```python
from build123d import *
from build123d import SkipClean  # not in build123d's __all__

# Parameters (mm, degrees)
F0_R      = 15
F1_DEPTH  = 67
F2_R      = 10
F3_DEPTH  = 11
F4_R      = 8.5
F5_DEPTH  = 1.9
F6_R      = 6.5
F7_DEPTH  = 2.1
F9_DEPTH  = 2
F10_W     = 1.5
F10_H     = 7
F11_DEPTH = 7
F13_DEPTH = 9.0692195411
F15_DEPTH = 25
F16_R     = 13.5
F17_DEPTH = 58.88


with BuildPart() as f1:
    # F0 (on Front) → F1 (new body)
    with BuildSketch(Plane.XZ):
        Circle(F0_R)
    extrude(amount=F1_DEPTH)

    # F2 (on face) → F3 (join)
    with BuildSketch(Plane.XZ.offset(67)):
        with Locations((-3.3, 0)):
            Circle(F2_R)
    extrude(amount=F3_DEPTH)

    # F4 (on face) → F5 (join)
    with BuildSketch(Plane.XZ.offset(78)):
        with Locations((-3.3, 0)):
            Circle(F4_R)
    extrude(amount=F5_DEPTH)

    # F6 (on face) → F7 (cut)
    with BuildSketch(Plane.XZ.offset(79.9)):
        with Locations((-3.3, 0)):
            Circle(F6_R)
    extrude(amount=-F7_DEPTH, mode=Mode.SUBTRACT)

    # F8 (on face) → F9 (cut)
    with BuildSketch(Plane.XZ.offset(77.8)):
        with BuildLine():
            ThreePointArc((-2.3067915896, -5), (1.2287423164, -3.5355339059), (2.6932084104, 0))
            ThreePointArc((2.6932084104, 0), (1.2757387706, 3.4879042731), (-2.1729820769, 4.9982091807))
            Line((-2.1729820769, 4.9982091807), (-2.3067915896, -5))
        make_face()
    extrude(amount=-F9_DEPTH, mode=Mode.SUBTRACT)

    # F10 (on face) → F11 (join)
    with BuildSketch(Plane.XZ.offset(77.8)):
        with Locations((-6.6817804589, 0.1302052614)):
            Rectangle(F10_W, F10_H)
    extrude(amount=F11_DEPTH)

    # F12 (on face) → F13 (cut, through all)
    with BuildSketch(Plane.YZ.offset(-5.9317804589)):
        Polygon((-77.8, -3.3697947386), (-84.8, 0.1302052614), (-84.8, -3.3697947386), align=None)
    with SkipClean():  # cleaning this boolean's faces spoils the solid; the shape is the same uncleaned
        extrude(amount=-F13_DEPTH, mode=Mode.SUBTRACT)

    # F14 (on face) → F15 (cut)
    with BuildSketch(Plane.YZ.offset(-5.9317804589)):
        Polygon((-84.8, 3.6302052614), (-84.8, 0.1302052614), (-77.8, 3.6302052614), align=None)
    extrude(amount=-F15_DEPTH, mode=Mode.SUBTRACT)

    # F16 (on face) → F17 (cut)
    with BuildSketch(Plane(origin=(0, 0, 0), x_dir=(-1, 0, 0), z_dir=(0, 1, 0))):
        Circle(F16_R)
    extrude(amount=-F17_DEPTH, mode=Mode.SUBTRACT)


solid = f1.part
```
Geometry: final body of the model. Coordinates: model frame, mm. A direction names the side the tool comes from. Give positions to 0.01 mm unless a question says otherwise; leave off trailing zeros. Order: outer loops, then holes, each group sorted by start corner. A loop starts at its lowest first (then second) coordinate and runs counter-clockwise, first axis right, second up. Notation, with made-up numbers: (-35.75, 10.5) -> (8.25, 10.5) arc R10 ccw to (8.25, 17.5) -> close; hole circle Ø10 at (-32.75, 42.25). An arc over 180 degrees is marked (long way). Write each question's results on one line, items separated by ' | '. Start each with the question number.
1) Line query: line 1 (X direction, y = -79.4, z = 0); line 2 (Y direction, x = -4, z = 11.5); line 3 (Y direction, x = -1.75, z = 3). Output: solid intervals per line, ascending. Write a range as from..to.
2) Section B-B (x = 4). Return loops of the section in (y, z), then the cut area to 3 significant figures.
3) First-contact query: pin 1 (1 mm diameter, centred on x = -11, z = -8, fed in from -Y); pin 2 (1 mm diameter, centred on x = -4, y = -43, fed in from -Z); pin 3 (10 mm diameter, centred on x = -7.5, z = 6.5, fed in from -Y). Flat tips, straight axial feed; report the tip coordinate or a pass-through.
4) Set-up query: faces 1 (the flat face through (-11, -79.9, 0)), 2 (the cylindrical face through (2.93, -29.03, -13.18)), 3 (the cylindrical face through (-14.985, -33.031, 0.66)), 4 (the flat face through (-11.18, 0, 7.85)), 5 (the flat face through (-5.932, -80, 0)). Return all of +Z, -Z, +X, -X, +Y, -Y with unobstructed straight access to the full face (end or side cutting, diameter ignored); none if empty.
5) Section A-A (y = -23.5). Return loops of the section in (x, z), then the cut area to 3 significant figures.
6) Section C-C (x = -3.3). Return loops of the section in (y, z), then the cut area to 3 significant figures.
Calculated:
1) line 1: -11.8..-9.8, -7.43..-5.93, 3.2..5.2 | line 2: -67..-58.88 | line 3: -75.8..-58.88
2) outline: (-79.9, -4.35) -> (-78, -4.35) -> (-78, -6.83) -> (-67, -6.83) -> (-67, -14.46) -> (0, -14.46) -> (0, -12.89) -> (-58.88, -12.89) -> (-58.88, 12.89) -> (0, 12.89) -> (0, 14.46) -> (-67, 14.46) -> (-67, 6.83) -> (-78, 6.83) -> (-78, 4.35) -> (-79.9, 4.35) -> close | area: 586 mm2
3) pin 1: y = -67 | pin 2: z = -14.59 | pin 3: y = -82.06
4) face 1: +Z, -Z, -X, -Y | face 2: +Y | face 3: +Y, -Y | face 4: +Z, -Z, +X, -X, +Y | face 5: -Y
5) outline: circle Ø30 at (0, 0); hole circle Ø27 at (0, 0) | area: 134 mm2
6) outline: (-79.9, -8.5) -> (-78, -8.5) -> (-78, -10) -> (-67, -10) -> (-67, -14.63) -> (0, -14.63) -> (0, -13.09) -> (-58.88, -13.09) -> (-58.88, 13.09) -> (0, 13.09) -> (0, 14.63) -> (-67, 14.63) -> (-67, 10) -> (-78, 10) -> (-78, 8.5) -> (-79.9, 8.5) -> (-79.9, 6.5) -> (-77.8, 6.5) -> (-77.8, -6.5) -> (-79.9, -6.5) -> close | area: 644 mm2
